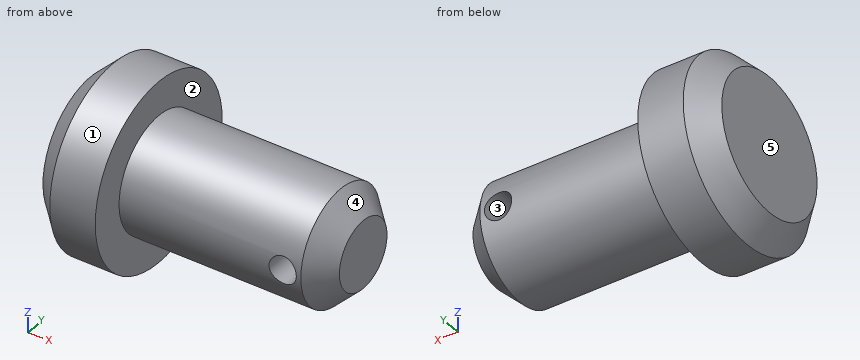
from build123d import *

# Parameters (mm, degrees)
SKETCH_2_W = 6
SKETCH_2_H = 84


with BuildPart() as part:
    # 草圖1 → 迴轉1 (revolve)
    with BuildSketch(Plane.XY, mode=Mode.PRIVATE) as revolve_1_sk:
        Polygon((0, 0), (-120, 0), (-120, 30), (-110, 40), (-90, 40), (-90, 25), (-10, 25), (0, 15), align=None)
    revolve(revolve_1_sk.sketch.rotate(Axis((0, 0, 0), (-1, 0, 0)), 90), axis=Axis((0, 0, 0), (-1, 0, 0)))

    # 草圖2 → 迴轉2 (revolve, cut)
    with BuildSketch(Plane.XY, mode=Mode.PRIVATE) as cut_revolve_2_sk:
        with Locations((-21, -9)):
            Rectangle(SKETCH_2_W, SKETCH_2_H)
    revolve(cut_revolve_2_sk.sketch.rotate(Axis((-18, -51, 0), (0, 1, 0)), 270), axis=Axis((-18, -51, 0), (0, 1, 0)), mode=Mode.SUBTRACT)


solid = part.part
Verification items for the finished model (mm, model axes). Face numbers are marked on the shaded views. A direction names the side the tool comes from. Coordinates: 2 decimals unless noted, no trailing zeros. Write each loop counter-clockwise with the first axis right and the second up, starting at its lowest first coordinate (ties: lowest second). Pieces come first, ordered by that corner, then holes. Notation, with made-up numbers: M 3.5,84.5 L 33.5,84.5 A16 cw 33.5,95.5 Z; hole C -24,66.5 d8. An arc over 180 degrees is marked long. One line per question, with ' | ' between items.
1) Sectioned sample at B-B on y = 0. Record the cut outline in (x, z).
Solutions:
outline: M -120,-30 L -110,-40 L -90,-40 L -90,-25 L -10,-25 L 0,-15 L 0,15 L -10,25 L -90,25 L -90,40 L -110,40 L -120,30 Z; hole C -18,0 d12
2) Material ranges on L1, parallel to X at y = 1, z = 0; L2, parallel to X at y = -6.5, z = -27; L3, parallel to Z at x = -18, y = -3, recorded low to high.
Solutions:
L1: -120 to -24, -12 to 0 | L2: -120 to -90 | L3: -24.82 to -6, 6 to 24.82
3) Access from +Z, -Z, +X, -X, +Y, -Y to the whole of each face (thin tool, end or side, straight path). Record for the marked faces 1 and 2.
Solutions:
face 1: +X, -X | face 2: +X
4) Sectioned sample at A-A on z = 0. Record the cut outline in (x, y), then the cut area to 3 significant figures.
Solutions:
outline: M -120,-30 L -110,-40 L -90,-40 L -90,-25 L -24,-25 L -24,25 L -90,25 L -90,40 L -110,40 L -120,30 Z; M -12,-25 L -10,-25 L 0,-15 L 0,15 L -10,25 L -12,25 Z | area: 6,100 mm^2
5) Release check for a two-part mould opening along X. For the marked faces 3, 4 and 5 record: +X half, -X half, draft (parallel to the pull), parting line (faces both ways), or undercut.
Solutions:
face 3: undercut | face 4: +X half | face 5: -X half
6) Sectioned sample at D-D on x = -33.5. Record the cut outline in (y, z).
Solutions:
outline: C 0,0 d50
7) Depth check by flat-ended pin: pin 1 Ø15.5 at (x, z) = (-18, 0) entering from -Y; pin 2 Ø3 at (y, z) = (-13, -21.5) entering from +X; pin 3 Ø3 at (x, z) = (-47.5, -19.5) entering from -Y. Enter the tip coordinate at first touch or a pass-through.
Solutions:
pin 1: y = -25 | pin 2: x = -8.62 | pin 3: y = -17.35
8) Sectioned sample at C-C on x = -92.5. Record the cut outline in (y, z), then the cut area to 3 significant figures.
Solutions:
outline: C 0,0 d80 | area: 5,030 mm^2
